from build123d import *

# Parameters (mm, degrees)
SKETCH2_R           = 1.610129379
SKETCH2_R_2         = 1.66029091
SKETCH2_R_3         = 1.791193395
SKETCH2_R_4         = 1.600916599
BOSS_EXTRUDE1_DEPTH = 1.5
SKETCH3_W           = 19.081191899
SKETCH3_H           = 5.85855086
SKETCH3_W_2         = 19.299887508
SKETCH3_H_2         = 5.534917291
BOSS_EXTRUDE2_DEPTH = 0.5
SKETCH4_W           = 24.601924878
SKETCH4_H           = 24.16573396
SKETCH4_W_2         = 21.926940144
SKETCH4_H_2         = 21.538176574
BOSS_EXTRUDE3_DEPTH = 1


with BuildPart() as part:
    # Sketch2 → Boss-Extrude1 (new body)
    with BuildSketch(Plane(origin=(0, 0, 0), x_dir=(1, 0, 0), z_dir=(0, 1, 0))):
        with BuildLine():
            Line((8.404082058, 20), (47.595917942, 20))
            ThreePointArc((47.595917942, 20), (56, 0), (47.595917942, -20))
            Line((47.595917942, -20), (8.404082058, -20))
            ThreePointArc((8.404082058, -20), (0, 0), (8.404082058, 20))
        make_face()
        with Locations(Location((11.087651709, 17.343003221, 0), (0, 0, 270))):
            Circle(SKETCH2_R, mode=Mode.SUBTRACT)
        with Locations(Location((11.087651709, -16.98750612, 0), (0, 0, 270))):
            Circle(SKETCH2_R_2, mode=Mode.SUBTRACT)
        with Locations(Location((45.262584723, -16.98750612, 0), (0, 0, 270))):
            Circle(SKETCH2_R_3, mode=Mode.SUBTRACT)
        with Locations(Location((45.262584723, 17.343003221, 0), (0, 0, 270))):
            Circle(SKETCH2_R_4, mode=Mode.SUBTRACT)
    extrude(amount=BOSS_EXTRUDE1_DEPTH)

    # Sketch3 → Boss-Extrude2 (add)
    with BuildSketch(Plane(origin=(0, 1.5, 0), x_dir=(1, 0, 0), z_dir=(0, 1, 0))):
        with Locations((31.069199174, 22.92927543)):
            Rectangle(SKETCH3_W, SKETCH3_H)
        with Locations((25.055069922, -22.767458645)):
            Rectangle(SKETCH3_W_2, SKETCH3_H_2)
    extrude(amount=-BOSS_EXTRUDE2_DEPTH)

    # Sketch4 → Boss-Extrude3 (add)
    with BuildSketch(Plane(origin=(0, 1.5, 0), x_dir=(1, 0, 0), z_dir=(0, 1, 0))):
        with Locations((28, 0)):
            Rectangle(SKETCH4_W, SKETCH4_H)
        with Locations((28, 0)):
            Rectangle(SKETCH4_W_2, SKETCH4_H_2, mode=Mode.SUBTRACT)
    extrude(amount=BOSS_EXTRUDE3_DEPTH)


solid = part.part
Verification items for the finished model (mm, model axes). A direction names the side the tool comes from. Coordinates: 2 decimals unless noted, no trailing zeros. Order: outer loops, then holes, each group sorted by start corner. A loop starts at its lowest first (then second) coordinate and runs counter-clockwise, first axis right, second up. Notation, with made-up numbers: M -35,22.5 L 18,22.5 A16 ccw 18,39.5 Z; hole C -4.75,1 d5. An arc over 180 degrees is marked long. Return JSON: item names as keys, results as strings.
1) Cross-section at D-D, the plane z = -2. Record the boundary of the cut face in (x, y), and give its area (3 significant figures).
Answer list:
{"outline": "M 0.07,0 L 55.93,0 L 55.93,1.5 L 40.3,1.5 L 40.3,2.5 L 38.96,2.5 L 38.96,1.5 L 17.04,1.5 L 17.04,2.5 L 15.7,2.5 L 15.7,1.5 L 0.07,1.5 Z", "area": "86.5 mm2"}
2) Gauge pin test, flat ends, axial feed: pin 1 (4.5 mm diameter, centred on x = 27.5, z = 23.5, fed in from -Y); pin 2 (3 mm diameter, centred on x = 45.26, z = 16.99, fed in from -Y); pin 3 (0.6 mm diameter, centred on y = 1, z = -22, fed in from -X); pin 4 (1.5 mm diameter, centred on y = 0.5, z = 14, fed in from +X). Record the tip position at first contact, or that the pin passes through.
Answer list:
{"pin 1": "y = 1", "pin 2": "through", "pin 3": "x = 21.53", "pin 4": "x = 52.67"}
3) Access from +Z, -Z, +X, -X, +Y, -Y to the whole of each face (thin tool, end or side, straight path). Record for faces 4 (the cylindrical face through (10.11, 0.74, -18.62)), 5 (the flat face through (31, 1, -23)), 6 (the flat face through (25, 1, 23)).
Answer list:
{"face 4": "+Y, -Y", "face 5": "-Z, +X, -X, -Y", "face 6": "+Z, +X, -X, -Y"}
4) Thickness scan on L1, parallel to X at y = 1.85, z = -9.5; L2, parallel to Z at x = 34, y = 2; L3, parallel to Y at x = 42.5, z = -4. Record the ranges inside material, lowest first. Write a range as [from, to].
Answer list:
{"L1": "[15.7, 17.04], [38.96, 40.3]", "L2": "[-12.08, -10.77], [10.77, 12.08]", "L3": "[0, 1.5]"}
5) Cross-section at B-B, the plane x = 24.5. Record the boundary of the cut face in (y, z), and give its area (3 significant figures).
Answer list:
{"outline": "M 0,-20 L 1,-20 L 1,-25.86 L 1.5,-25.86 L 1.5,-12.08 L 2.5,-12.08 L 2.5,-10.77 L 1.5,-10.77 L 1.5,10.77 L 2.5,10.77 L 2.5,12.08 L 1.5,12.08 L 1.5,25.53 L 1,25.53 L 1,20 L 0,20 Z", "area": "68.3 mm2"}
6) Cross-section at A-A, the plane y = 1.95. Record the boundary of the cut face in (x, z), and give its area (3 significant figures).
Answer list:
{"outline": "M 15.7,-12.08 L 40.3,-12.08 L 40.3,12.08 L 15.7,12.08 Z; hole M 17.04,-10.77 L 38.96,-10.77 L 38.96,10.77 L 17.04,10.77 Z", "area": "122 mm2"}
7) Cross-section at C-C, the plane z = 16. Record the boundary of the cut face in (x, y).
Answer list:
{"outline": "M 5.02,0 L 9.75,0 L 9.75,1.5 L 5.02,1.5 Z; M 12.42,0 L 43.77,0 L 43.77,1.5 L 12.42,1.5 Z; M 46.76,0 L 50.98,0 L 50.98,1.5 L 46.76,1.5 Z"}
8) Release check for a two-part mould opening along Z. For faces 1 (the cylindrical face through (0, 1, 0)), 2 (the flat face through (28, 1.5, 0)), 3 (the flat face through (28, 0, 0)) record: +Z half, -Z half, draft (parallel to the pull), parting line (faces both ways), or undercut.
Answer list:
{"face 1": "parting line", "face 2": "undercut", "face 3": "draft"}
